Check sheet for the modelled part. Datum: model origin and axes. Units: mm. Face numbers are marked on the shaded views. A direction names the side the tool comes from. Give positions to 0.01 mm unless a question says otherwise; leave off trailing zeros. Write each loop counter-clockwise with the first axis right and the second up, starting at its lowest first coordinate (ties: lowest second). Pieces come first, ordered by that corner, then holes. Notation, with made-up numbers: (-24, 62.5) -> (29, 62.5) arc R33 cw to (29, 92.5) -> close; hole circle Ø1 at (28.5, 86). An arc over 180 degrees is marked (long way). Use a Markdown table: item, result. Add a question column.
1. Gauge pin test, flat ends, axial feed: P1, Ø0.5, axis at x = 13, z = 2.5, coming from the +Y side; P2, Ø0.8, axis at x = 13.98, y = -7.6, coming from the +Z side; P3, Ø1, axis at y = -8, z = 2.5, coming from the -X side. Record the tip position at first contact, or that the pin passes through.
2. Cross-section at C-C (y = 5.5). Enter the section's corners in (x, z), then the cut area to 3 significant figures.
3. Set-up check for the marked faces 4, 5, 6, 7 and 8: record each of +Z, -Z, +X, -X, +Y, -Y from which the full face is reachable in a straight line by a thin tool's end or side.
4. Cross-section at A-A (y = 2.25). Enter the section's corners in (x, z).
5. Release check for a two-part mould opening along Y. For the marked faces 1, 2 and 3 record: released by +Y, released by -Y, zero draft, split by the parting line, or undercut.
6. Cross-section at D-D (x = -16.51). Enter the section's corners in (y, z) (3 decimals), then the cut area to 3 significant figures.
7. Scan lines: probe 1 along Y at (x, z) = (7, 2.05); probe 2 along Z at (x, y) = (12, -1.5); probe 3 along X at (y, z) = (-3.5, 1.1). Record each from-to range of solid material in increasing order. Write a range as [from, to].
8. Cross-section at B-B (x = -5). Enter the section's corners in (y, z), then the cut area to 3 significant figures.
from build123d import *

# Parameters (mm, degrees)
SKETCH_W          = 35.56
SKETCH_H          = 17.78
PAD_DEPTH         = 1.57
SKETCH001_R       = 0.635
POCKET_DEPTH      = 1.571
SKETCH002_W       = 2.2
SKETCH002_H       = 3
PAD001_DEPTH      = 2.5
FILLET_R          = 0.2
FILLET001_R       = 0.2
SKETCH003_W       = 5
SKETCH003_H       = 8.06
PAD002_DEPTH      = 2.9
FILLET002_R       = 0.2
FILLET003_R       = 0.2
SKETCH006_W       = 35.02
SKETCH006_H       = 2
PAD004_DEPTH      = 2
PAD004_DEPTH_BACK = 0.5


with BuildPart() as part:
    # Sketch → Pad (new body)
    with BuildSketch(Plane.XY):
        Rectangle(SKETCH_W, SKETCH_H)
    extrude(amount=PAD_DEPTH)

    # Sketch001 → Pocket (cut, through all)
    with BuildSketch(Plane.XY.offset(1.57)):
        with Locations((-16.51, 7.62)):
            Circle(SKETCH001_R)
        with Locations((-13.970001, 7.621845)):
            Circle(SKETCH001_R)
        with Locations((-11.430001, 7.623691)):
            Circle(SKETCH001_R)
        with Locations((-8.890002, 7.625536)):
            Circle(SKETCH001_R)
        with Locations((-6.350003, 7.627382)):
            Circle(SKETCH001_R)
        with Locations((-3.810003, 7.629227)):
            Circle(SKETCH001_R)
        with Locations((-1.270004, 7.631072)):
            Circle(SKETCH001_R)
        with Locations((1.269995, 7.632918)):
            Circle(SKETCH001_R)
        with Locations((3.809995, 7.634763)):
            Circle(SKETCH001_R)
        with Locations((6.349994, 7.636609)):
            Circle(SKETCH001_R)
        with Locations((8.889993, 7.638454)):
            Circle(SKETCH001_R)
        with Locations((11.429993, 7.640299)):
            Circle(SKETCH001_R)
        with Locations((13.969992, 7.642145)):
            Circle(SKETCH001_R)
        with Locations((16.509991, 7.64399)):
            Circle(SKETCH001_R)
        with Locations((-16.498928, -7.619996)):
            Circle(SKETCH001_R)
        with Locations((-13.958928, -7.618151)):
            Circle(SKETCH001_R)
        with Locations((-11.418929, -7.616305)):
            Circle(SKETCH001_R)
        with Locations((-8.87893, -7.61446)):
            Circle(SKETCH001_R)
        with Locations((-6.33893, -7.612614)):
            Circle(SKETCH001_R)
        with Locations((-3.798931, -7.610769)):
            Circle(SKETCH001_R)
        with Locations((-1.258932, -7.608924)):
            Circle(SKETCH001_R)
        with Locations((1.281068, -7.607078)):
            Circle(SKETCH001_R)
        with Locations((3.821067, -7.605233)):
            Circle(SKETCH001_R)
        with Locations((6.361066, -7.603387)):
            Circle(SKETCH001_R)
        with Locations((8.901066, -7.601542)):
            Circle(SKETCH001_R)
        with Locations((11.441065, -7.599697)):
            Circle(SKETCH001_R)
        with Locations((13.981064, -7.597851)):
            Circle(SKETCH001_R)
        with Locations((16.521064, -7.596006)):
            Circle(SKETCH001_R)
    extrude(amount=-POCKET_DEPTH, mode=Mode.SUBTRACT)

    # Sketch002 → Pad001 (new body)
    with BuildSketch(Plane.XY.offset(1.57)):
        with Locations((13.46, 0)):
            Rectangle(SKETCH002_W, SKETCH002_H)
    extrude(amount=PAD001_DEPTH)

    # Fillet
    fillet_edges = [part.edges().sort_by_distance(p)[0] for p in [
        (14.56, 1.5, 2.82),
        (14.56, -1.5, 2.82),
        (12.36, -1.5, 2.82),
        (12.36, 1.5, 2.82),
    ]]
    fillet(fillet_edges, radius=FILLET_R)

    # Fillet001
    fillet001_edges = [part.edges().sort_by_distance(p)[0] for p in [
        (13.46, 1.5, 4.07),
    ]]
    fillet(fillet001_edges, radius=FILLET001_R)

    # Sketch003 → Pad002 (new body)
    with BuildSketch(Plane.XY.offset(1.57)):
        with Locations((-15.98, 0)):
            Rectangle(SKETCH003_W, SKETCH003_H)
    extrude(amount=PAD002_DEPTH)

    # Fillet002
    fillet002_edges = [part.edges().sort_by_distance(p)[0] for p in [
        (-15.98, -4.03, 4.47),
        (-15.98, 4.03, 4.47),
    ]]
    fillet(fillet002_edges, radius=FILLET002_R)

    # Fillet003
    fillet003_edges = [part.edges().sort_by_distance(p)[0] for p in [
        (-18.48, 0, 4.47),
        (-13.48, 0, 4.47),
    ]]
    fillet(fillet003_edges, radius=FILLET003_R)

    # Sketch006 → Pad004 (new body, two sides)
    with BuildSketch(Plane.XY.offset(1.57)) as pad004_sk:
        with Locations((0, 7.62)):
            Rectangle(SKETCH006_W, SKETCH006_H)
    pad004 = extrude(amount=PAD004_DEPTH) + extrude(pad004_sk.sketch, amount=-PAD004_DEPTH_BACK)

    # Mirrored: Pad004 across Sketch006 H_Axis
    add(pad004.mirror(Plane(origin=(0, 0, 1.57), x_dir=(0, 0, 1), z_dir=(0, 1, 0))))


solid = part.part
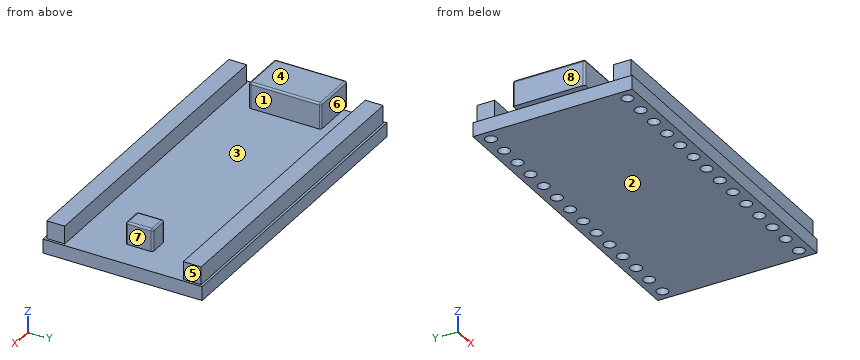
Worked answers:
| question | item | result |
|---|---|---|
| 1 | P1 | stops at y = 8.62 |
| 1 | P2 | stops at z = 3.57 |
| 1 | P3 | stops at x = -17.51 |
| 2 | outline | (-17.78, 0) -> (17.78, 0) -> (17.78, 1.57) -> (-17.78, 1.57) -> close |
| 2 | area | 55.8 mm² |
| 3 | face 4 | +Z, +X, -X, +Y, -Y |
| 3 | face 5 | +Z, +X, +Y, -Y |
| 3 | face 6 | +Z, +X, -X |
| 3 | face 7 | +Z, +X |
| 3 | face 8 | +Z, -Z, -X, +Y, -Y |
| 4 | outline | (-18.48, 1.57) -> (-17.78, 1.57) -> (-17.78, 0) -> (17.78, 0) -> (17.78, 1.57) -> (-13.48, 1.57) -> (-13.48, 4.27) arc R0.2 ccw to (-13.68, 4.47) -> (-18.28, 4.47) arc R0.2 ccw to (-18.48, 4.27) -> close |
| 5 | face 1 | undercut |
| 5 | face 2 | zero draft |
| 5 | face 3 | undercut |
| 6 | outline | (-8.89, 0) -> (-8.255, 0) -> (-8.255, 1.07) -> (-6.985, 1.07) -> (-6.985, 0) -> (6.985, 0) -> (6.985, 1.07) -> (8.255, 1.07) -> (8.255, 0) -> (8.89, 0) -> (8.89, 1.57) -> (8.62, 1.57) -> (8.62, 3.57) -> (6.62, 3.57) -> (6.62, 1.57) -> (4.03, 1.57) -> (4.03, 4.27) arc R0.2 ccw to (3.83, 4.47) -> (-3.83, 4.47) arc R0.2 ccw to (-4.03, 4.27) -> (-4.03, 1.57) -> (-6.62, 1.57) -> (-6.62, 3.57) -> (-8.62, 3.57) -> (-8.62, 1.57) -> (-8.89, 1.57) -> close |
| 6 | area | 56.6 mm² |
| 7 | probe 1 | y = [-8.62, -6.62], [6.62, 8.62] |
| 7 | probe 2 | z = [0, 1.57] |
| 7 | probe 3 | x = [-17.78, 17.78] |
| 8 | outline | (-8.89, 0) -> (8.89, 0) -> (8.89, 1.57) -> (8.62, 1.57) -> (8.62, 3.57) -> (6.62, 3.57) -> (6.62, 1.57) -> (-6.62, 1.57) -> (-6.62, 3.57) -> (-8.62, 3.57) -> (-8.62, 1.57) -> (-8.89, 1.57) -> close |
| 8 | area | 35.9 mm² |
